Geometry check sheet. Reference: drawing and pictorial views, mm from the part's lowest x, y, z. Round coordinates to 2 decimals unless told otherwise and drop trailing zeros. Write each loop counter-clockwise with the first axis right and the second up, starting at its lowest first coordinate (ties: lowest second). Pieces come first, ordered by that corner, then holes. Notation, with made-up numbers: M 22.5,25.5 L 38.5,25.5 A22 ccw 38.5,48.5 Z; hole C 14,64 d9. An arc over 180 degrees is marked long. One line per item, written item: value. Start each with the question number.
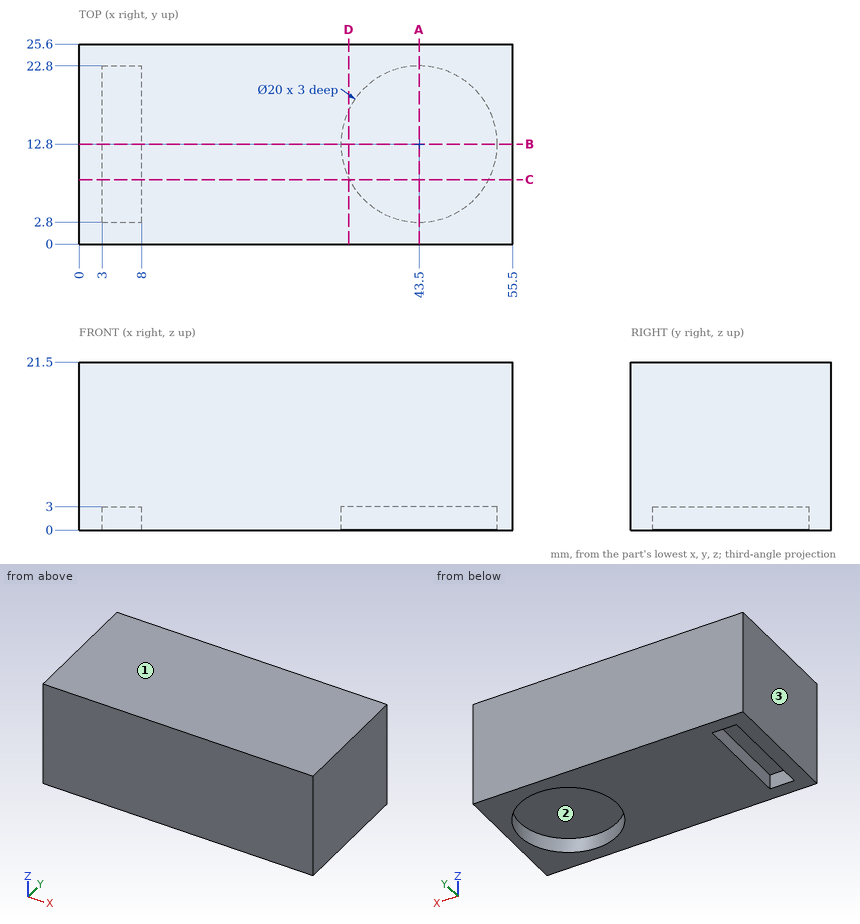
1) Cross-section at D-D (x = 34.5). Record the boundary of the cut face in (y, z).
2) Cross-section at A-A (x = 43.5). Record the boundary of the cut face in (y, z), then the cut area to 3 significant figures.
3) Mould release check, pull along X, two halves, no side actions. Record for the marked faces 1, 2 and 3: pulls with the +X half, pulls with the -X half, needs draft (parallel to the pull), parting line crosses it, or undercut.
4) Cross-section at C-C (y = 8.25). Record the boundary of the cut face in (x, z), then the cut area to 3 significant figures.
5) Cross-section at B-B (y = 12.8). Record the boundary of the cut face in (x, z).
6) Thickness scan on line 1 (Y direction, x = 43.5, z = 1.3); line 2 (X direction, y = 9.25, z = 2.5); line 3 (X direction, y = 18, z = 1.75). Record the ranges inside material, lowest first.
7) Gauge pin test, flat ends, axial feed: pin 1 Ø2.5 at (x, z) = (6, 1) entering from -Y; pin 2 Ø2.5 at (x, y) = (4.5, 14) entering from -Z. Record the tip position at first contact, or that the pin passes through.
Results below:
1. outline: M 0,0 L 8.44,0 L 8.44,3 L 17.16,3 L 17.16,0 L 25.6,0 L 25.6,21.5 L 0,21.5 Z
2. outline: M 0,0 L 2.8,0 L 2.8,3 L 22.8,3 L 22.8,0 L 25.6,0 L 25.6,21.5 L 0,21.5 Z
2. area: 490 mm²
3. face 1: needs draft
3. face 2: undercut
3. face 3: pulls with the -X half
4. outline: M 0,0 L 3,0 L 3,3 L 8,3 L 8,0 L 34.6,0 L 34.6,3 L 52.4,3 L 52.4,0 L 55.5,0 L 55.5,21.5 L 0,21.5 Z
4. area: 1,120 mm²
5. outline: M 0,0 L 3,0 L 3,3 L 8,3 L 8,0 L 33.5,0 L 33.5,3 L 53.5,3 L 53.5,0 L 55.5,0 L 55.5,21.5 L 0,21.5 Z
6. line 1: y = 0 to 2.8, 22.8 to 25.6
6. line 2: x = 0 to 3, 8 to 34.15, 52.85 to 55.5
6. line 3: x = 0 to 3, 8 to 34.96, 52.04 to 55.5
7. pin 1: stops at y = 0
7. pin 2: stops at z = 3
